Build history of the part. All positions in model axes, mm. Face numbers are marked on the shaded views. A direction names the side the tool comes from. Coordinates: 2 decimals unless noted, no trailing zeros. Loops run counter-clockwise (first coordinate to the right, second up) from the corner with the lowest first, then second, coordinate; pieces in that order, holes last. Notation, with made-up numbers: (59, 68) - (71, 68) arc R25 ccw to (71, 81) - close; hole circle Ø2 at (35.5, -26). An arc over 180 degrees is marked (long way). One line per item, written item: value.
```python
from build123d import *

# Parameters (mm, degrees)
SKETCH_1_R          = 9.5
EXTRUDE_1_DEPTH     = 85
SKETCH_2_R          = 15
EXTRUDE_2_DEPTH     = 10
SKETCH_3_R          = 19.5
EXTRUDE_3_DEPTH     = 13
SKETCH_4_R          = 15
EXTRUDE_4_DEPTH     = 29
CHAMFER_1_SIZE      = 1
SKETCH_5_R          = 7.5
CUT_EXTRUDE_1_DEPTH = 140.747987463


with BuildPart() as part:
    # Эскиз1 → Бобышка-Вытянуть1 (new body)
    with BuildSketch(Plane.XY):
        Circle(SKETCH_1_R)
    extrude(amount=EXTRUDE_1_DEPTH)

    # Эскиз2 → Бобышка-Вытянуть2 (add)
    with BuildSketch(Plane.XY.offset(85)):
        Circle(SKETCH_2_R)
    extrude(amount=EXTRUDE_2_DEPTH)

    # Эскиз3 → Бобышка-Вытянуть3 (add)
    with BuildSketch(Plane.XY.offset(95)):
        with Locations(Location((0, 0, 0), (0, 0, 180))):
            Circle(SKETCH_3_R)
    extrude(amount=EXTRUDE_3_DEPTH)

    # Эскиз4 → Бобышка-Вытянуть4 (add)
    with BuildSketch(Plane.XY.offset(108)):
        Circle(SKETCH_4_R)
    extrude(amount=EXTRUDE_4_DEPTH)

    # Фаска1
    chamfer_1_edges = [part.edges().sort_by_distance(p)[0] for p in [
        (-15, 0, 137),
    ]]
    chamfer(chamfer_1_edges, length=CHAMFER_1_SIZE)

    # Эскиз5 → Вырез-Вытянуть1 (cut, through all)
    with BuildSketch(Plane(origin=(0, 0, 0), x_dir=(-1, 0, 0), z_dir=(0, 0, -1))):
        Circle(SKETCH_5_R)
    extrude(amount=-CUT_EXTRUDE_1_DEPTH, mode=Mode.SUBTRACT)


solid = part.part
```
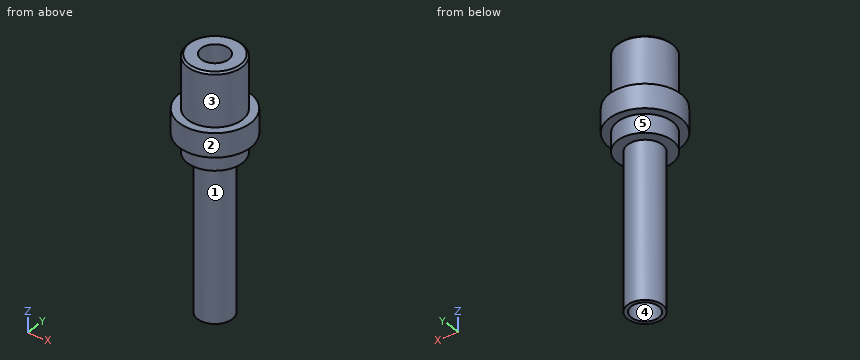
Item 1: Cut at D-D, the plane z = 98.5. Write the cut outline in (x, y).
Check result:
outline: circle Ø39 at (0, 0); hole circle Ø15 at (0, 0)
Item 2: Probe probe 1 along Y at (x, z) = (0, 52); probe 2 along Y at (x, z) = (0, 98); probe 3 along Z at (x, y) = (-9, -9). List the from-to ranges inside material, lowest first. Write a range as from..to.
Check result:
probe 1: y = -9.5..-7.5, 7.5..9.5
probe 2: y = -19.5..-7.5, 7.5..19.5
probe 3: z = 85..137
Item 3: Cut at C-C, the plane z = 51. Write the cut outline in (x, y), then the cut area to 3 significant figures.
Check result:
outline: circle Ø19 at (0, 0); hole circle Ø15 at (0, 0)
area: 107 mm^2
Item 4: Cut at A-A, the plane y = 0. Write the cut outline in (x, z).
Check result:
outline: (-19.5, 95) - (-15, 95) - (-15, 85) - (-9.5, 85) - (-9.5, 0) - (-7.5, 0) - (-7.5, 137) - (-14, 137) - (-15, 136) - (-15, 108) - (-19.5, 108) - close; (7.5, 0) - (9.5, 0) - (9.5, 85) - (15, 85) - (15, 95) - (19.5, 95) - (19.5, 108) - (15, 108) - (15, 136) - (14, 137) - (7.5, 137) - close
Item 5: Pull direction Y, two halves, no side cores. Call the marked faces 4 and 5: released by +Y, released by -Y, zero draft, split by the parting line, or undercut.
Check result:
face 4: undercut
face 5: split by the parting line
Item 6: Drop flat-ended pins along their axis: P1, Ø4, axis at x = 11, y = 12.5, coming from the +Z side; P2, Ø1.5, axis at y = -5, z = 29, coming from the +X side; P3, Ø12, axis at x = 10, z = 14.5, coming from the -Y side. Give the stop position or say it passes through.
Check result:
P1: stops at z = 136.35
P2: stops at x = 8.5
P3: stops at y = -8.62
Item 7: Tool access for the marked faces 1, 2 and 3: list every direction of +Z, -Z, +X, -X, +Y, -Y with a clear straight run to the whole face (end or side of a thin tool).
Check result:
face 1: -Z
face 2: +Z, -Z
face 3: +Z
